For this review, take the finished solid that the model builds, in its own axes (mm). Give positions to 0.01 mm unless a question says otherwise; leave off trailing zeros. Loops run counter-clockwise (first coordinate to the right, second up) from the corner with the lowest first, then second, coordinate; pieces in that order, holes last.
Autodesk Inventor part; units mm, degrees
ref_plane "YZ Plane" through (0, 0, 0) normal (1, 0, 0) x (0, 1, 0)
ref_plane "XZ Plane" through (0, 0, 0) normal (0, 1, 0) x (-1, 0, 0)
ref_plane "XY Plane" through (0, 0, 0) normal (0, 0, 1) x (1, 0, 0)
sketch "Sketch1" plane through (0, 0, 0) normal (0, 1, 0) x (-1, 0, 0)
  line L0 (900, 40) -> (-900, 40)
  line L1 (-900, 40) -> (-900, -40)
  line L2 (-900, -40) -> (900, -40)
  line L3 (900, -40) -> (900, 40)
  line L4 (900, 40) -> (-900, -40) construction
  line L5 (700, 40) -> (746.188, -40)
  line L6 (0, 40) -> (0, -40) construction
  line L7 (-700, 40) -> (-746.188, -40)
  point P0 (0, 0)
  point P1 (0, 0)
  dimension "d0" = 80
  dimension "d1" = 1800
  dimension "d3" = 120
  dimension "d6" = 700
  dimension "d7" = 120
  dimension "d8" = 700
extrude "Plate1" add sketch "Sketch1" along normal mid plane 3 contours L5 L2 L7 L0
sketch "Sketch2" plane through (0, -1.5, 0) normal (0, -1, 0) x (1, 0, 0)
  line L0 (-1.6, -40) -> (1.6, -40)
  line L1 (1.6, -40) -> (1.6, 1)
  line L2 (1.6, 1) -> (-1.6, 1)
  line L3 (-1.6, 1) -> (-1.6, -40)
  line L4 (746.188, -40) -> (-746.188, -40)
  point P0 (0, 0)
  point P1 (0, -40)
  dimension "d9" = 3.2
  dimension "d10" = 41
extrude "Extrusion1" cut sketch "Sketch2" against normal through all
pattern_linear "Rectangular Pattern1" count 5 spacing 240 along (1, 0, 0) of "Extrusion1" first direction both ways yes
equation "\"d7\" = d3"
equation "\"d8\" = d6"
equation "\"d2\" = Thickness"
equation "\"BendReliefWidth\" = Thickness"
equation "\"BendReliefDepth\" = 0.5 * Thickness"
equation "\"CornerReliefSize\" = 4 * Thickness"
equation "\"MinimumRemnant\" = 2 * Thickness"
equation "\"TransitionRadius\" = BendRadius"
equation "\"JacobiRadiusSize\" = BendRadius"
equation "\"GapSize\" = Thickness"
properties part number "MSC 201 GRID" material "Stainless Steel"
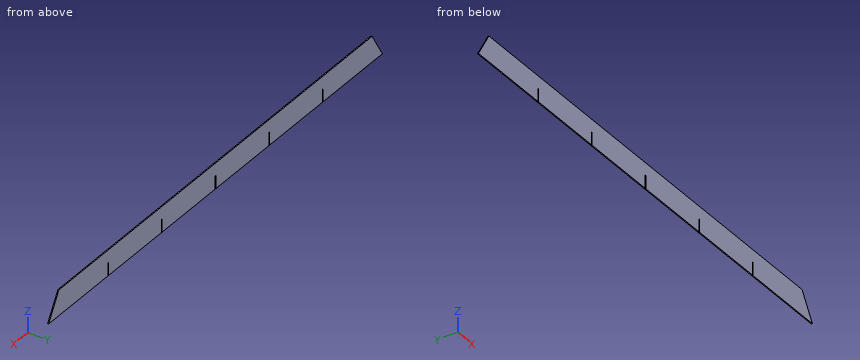
Q1. Consider section B-B on y = 0.2. Give the boundary of the cut face in (x, z).
Answers:
outline: (-746.19, -40) - (-481.6, -40) - (-481.6, 1) - (-478.4, 1) - (-478.4, -40) - (-241.6, -40) - (-241.6, 1) - (-238.4, 1) - (-238.4, -40) - (-1.6, -40) - (-1.6, 1) - (1.6, 1) - (1.6, -40) - (238.4, -40) - (238.4, 1) - (241.6, 1) - (241.6, -40) - (478.4, -40) - (478.4, 1) - (481.6, 1) - (481.6, -40) - (746.19, -40) - (700, 40) - (-700, 40) - close
Q2. Consider section A-A on z = -23.5. Give the boundary of the cut face in (x, y).
Answers:
outline: (-736.66, -1.5) - (-481.6, -1.5) - (-481.6, 1.5) - (-736.66, 1.5) - close; (-478.4, -1.5) - (-241.6, -1.5) - (-241.6, 1.5) - (-478.4, 1.5) - close; (-238.4, -1.5) - (-1.6, -1.5) - (-1.6, 1.5) - (-238.4, 1.5) - close; (1.6, -1.5) - (238.4, -1.5) - (238.4, 1.5) - (1.6, 1.5) - close; (241.6, -1.5) - (478.4, -1.5) - (478.4, 1.5) - (241.6, 1.5) - close; (481.6, -1.5) - (736.66, -1.5) - (736.66, 1.5) - (481.6, 1.5) - close
Q3. For pin 1 Ø1.5 at (x, y) = (-479.5, -0.5) entering from -Z; pin 2 Ø1 at (y, z) = (-1, -16.5) entering from +X; pin 3 Ø0.9 at (y, z) = (0.5, -19) entering from -X, all flat-tipped, find the tip position at first contact; note any pin that passes through.
Answers:
pin 1: stops at z = 1
pin 2: stops at x = 732.91
pin 3: stops at x = -734.32
Q4. For probe 1 along X at (y, z) = (-1.4, -17); probe 2 along X at (y, z) = (0.3, -6.5); probe 3 along X at (y, z) = (1.1, 9), list the stretches that pass through material, from the lowest coordinate up.
Answers:
probe 1: x = -732.91 to -481.6, -478.4 to -241.6, -238.4 to -1.6, 1.6 to 238.4, 241.6 to 478.4, 481.6 to 732.91
probe 2: x = -726.85 to -481.6, -478.4 to -241.6, -238.4 to -1.6, 1.6 to 238.4, 241.6 to 478.4, 481.6 to 726.85
probe 3: x = -717.9 to 717.9
